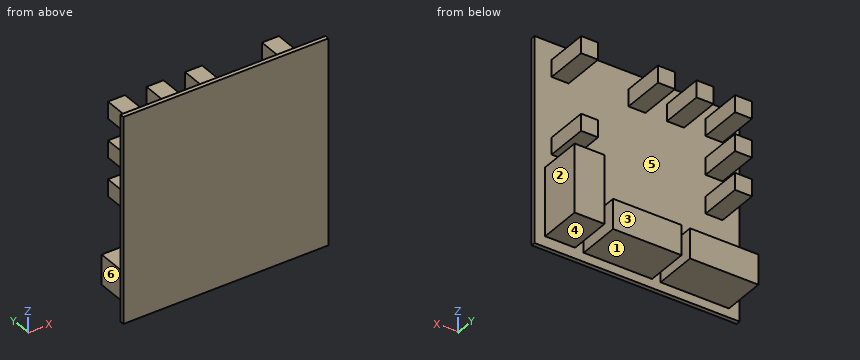
from build123d import *

# Parameters (mm, degrees)
SKETCH1_W              = 1.01
SKETCH1_H              = 1.01
BOSS_EXTRUDE1_DEPTH    = 2.54
BOSS_EXTRUDE1_2_DEPTH  = 2.54
BOSS_EXTRUDE1_3_DEPTH  = 2.54
BOSS_EXTRUDE1_4_DEPTH  = 2.54
BOSS_EXTRUDE1_5_DEPTH  = 2.54
BOSS_EXTRUDE1_6_DEPTH  = 2.54
BOSS_EXTRUDE1_7_DEPTH  = 2.54
SKETCH1_W_2            = 1.778
SKETCH1_H_2            = 4.064
BOSS_EXTRUDE1_8_DEPTH  = 2.54
SKETCH1_W_3            = 4.064
SKETCH1_H_3            = 1.778
BOSS_EXTRUDE1_9_DEPTH  = 2.54
BOSS_EXTRUDE1_10_DEPTH = 2.54
SKETCH3_W              = 12.192
SKETCH3_H              = 12.192
BOSS_EXTRUDE2_DEPTH    = 0.254


with BuildPart() as part:
    # Sketch1 (on Top Plane) → Boss-Extrude1 (new body)
    with BuildSketch(Plane(origin=(0, 0, 0), x_dir=(1, 0, 0), z_dir=(0, 1, 0))):
        with Locations((1.52, 1.52)):
            Rectangle(SKETCH1_W, SKETCH1_H)
    extrude(amount=BOSS_EXTRUDE1_DEPTH)



with BuildPart() as body_2:
    # Sketch1 (on Top Plane) → Boss-Extrude1 2 (new body)
    with BuildSketch(Plane(origin=(0, 0, 0), x_dir=(1, 0, 0), z_dir=(0, 1, 0))):
        with Locations((1.52, 6.096)):
            Rectangle(SKETCH1_W, SKETCH1_H)
    extrude(amount=BOSS_EXTRUDE1_2_DEPTH)


with BuildPart() as body_3:
    # Sketch1 (on Top Plane) → Boss-Extrude1 3 (new body)
    with BuildSketch(Plane(origin=(0, 0, 0), x_dir=(1, 0, 0), z_dir=(0, 1, 0))):
        with Locations((1.52, 3.81)):
            Rectangle(SKETCH1_W, SKETCH1_H)
    extrude(amount=BOSS_EXTRUDE1_3_DEPTH)


with BuildPart() as body_4:
    # Sketch1 (on Top Plane) → Boss-Extrude1 4 (new body)
    with BuildSketch(Plane(origin=(0, 0, 0), x_dir=(1, 0, 0), z_dir=(0, 1, 0))):
        with Locations((10.67, 1.52)):
            Rectangle(SKETCH1_W, SKETCH1_H)
    extrude(amount=BOSS_EXTRUDE1_4_DEPTH)


with BuildPart() as body_5:
    # Sketch1 (on Top Plane) → Boss-Extrude1 5 (new body)
    with BuildSketch(Plane(origin=(0, 0, 0), x_dir=(1, 0, 0), z_dir=(0, 1, 0))):
        with Locations((6.1, 1.52)):
            Rectangle(SKETCH1_W, SKETCH1_H)
    extrude(amount=BOSS_EXTRUDE1_5_DEPTH)


with BuildPart() as body_6:
    # Sketch1 (on Top Plane) → Boss-Extrude1 6 (new body)
    with BuildSketch(Plane(origin=(0, 0, 0), x_dir=(1, 0, 0), z_dir=(0, 1, 0))):
        with Locations((3.81, 1.52)):
            Rectangle(SKETCH1_W, SKETCH1_H)
    extrude(amount=BOSS_EXTRUDE1_6_DEPTH)


with BuildPart() as body_7:
    # Sketch1 (on Top Plane) → Boss-Extrude1 7 (new body)
    with BuildSketch(Plane(origin=(0, 0, 0), x_dir=(1, 0, 0), z_dir=(0, 1, 0))):
        with Locations((10.67, 6.096)):
            Rectangle(SKETCH1_W, SKETCH1_H)
    extrude(amount=BOSS_EXTRUDE1_7_DEPTH)


with BuildPart() as body_8:
    # Sketch1 (on Top Plane) → Boss-Extrude1 8 (new body)
    with BuildSketch(Plane(origin=(0, 0, 0), x_dir=(1, 0, 0), z_dir=(0, 1, 0))):
        with Locations((10.67, 9.525)):
            Rectangle(SKETCH1_W_2, SKETCH1_H_2)
    extrude(amount=BOSS_EXTRUDE1_8_DEPTH)


with BuildPart() as body_9:
    # Sketch1 (on Top Plane) → Boss-Extrude1 9 (new body)
    with BuildSketch(Plane(origin=(0, 0, 0), x_dir=(1, 0, 0), z_dir=(0, 1, 0))):
        with Locations((2.667, 10.769327267)):
            Rectangle(SKETCH1_W_3, SKETCH1_H_3)
    extrude(amount=BOSS_EXTRUDE1_9_DEPTH)


with BuildPart() as body_10:
    # Sketch1 (on Top Plane) → Boss-Extrude1 10 (new body)
    with BuildSketch(Plane(origin=(0, 0, 0), x_dir=(1, 0, 0), z_dir=(0, 1, 0))):
        with Locations((7.239, 10.769327267)):
            Rectangle(SKETCH1_W_3, SKETCH1_H_3)
    extrude(amount=BOSS_EXTRUDE1_10_DEPTH)


with BuildPart() as part_1:
    add(part.part)

    add(body_2.part)  # Boss-Extrude2 merges body 2

    add(body_3.part)  # Boss-Extrude2 merges body 3

    add(body_4.part)  # Boss-Extrude2 merges body 4

    add(body_5.part)  # Boss-Extrude2 merges body 5

    add(body_6.part)  # Boss-Extrude2 merges body 6

    add(body_7.part)  # Boss-Extrude2 merges body 7

    add(body_8.part)  # Boss-Extrude2 merges body 8

    add(body_9.part)  # Boss-Extrude2 merges body 9

    add(body_10.part)  # Boss-Extrude2 merges body 10
    # Sketch3 → Boss-Extrude2 (add)
    with BuildSketch(Plane.XZ):
        with Locations((6.096, -6.096)):
            Rectangle(SKETCH3_W, SKETCH3_H)
    extrude(amount=BOSS_EXTRUDE2_DEPTH)


solid = part_1.part
The model under review builds one solid part; all positions refer to its coordinate system, in mm. Face numbers are marked on the shaded views. A direction names the side the tool comes from. Round coordinates to 2 decimals unless told otherwise and drop trailing zeros. Loops run counter-clockwise (first coordinate to the right, second up) from the corner with the lowest first, then second, coordinate; pieces in that order, holes last. Notation, with made-up numbers: M -3.5,-1.75 L 2.5,-1.75 A17 cw 2.5,8.25 Z; hole C -15,9.25 d6. An arc over 180 degrees is marked long. Answer as CSV lines item,"result". Start each with the question number.
Item 1: Mouldability with a two-part tool opening along X and no side actions: class the marked faces 4, 5 and 6 as released by +X, released by -X, zero draft, split by the parting line, or undercut.
Item 2: Consider section B-B (x = 4.5). Write out the cut boundary in (y, z), then the cut area to 3 significant figures.
Item 3: For the marked faces 1, 2 and 3, list the 3-axis set-ups (+Z, -Z, +X, -X, +Y, -Y) from which the entire face can be reached by the end or side of a thin tool; tool diameter is ignored.
Item 4: Consider section D-D (z = -8). Write out the cut boundary in (x, y), then the cut area to 3 significant figures.
Item 5: Insertion check: P1, Ø1.1, axis at y = 1, z = -1.5, coming from the -X side (3 decimals); P2, Ø0.9, axis at y = 1.5, z = -10.5, coming from the -X side (3 decimals); P3, Ø0.5, axis at x = 1.5, y = 2, coming from the +Z side (3 decimals). Each pin has a flat end and moves straight along its axis. Give the tip position at first contact, or say it passes through.
Item 6: Consider section C-C (y = 1.35). State how many separate pieces and enclosed holes the cut face has, then the cut area to 3 significant figures.
Item 7: Wall thickness on line 1 (Z direction, x = 1.25, y = 2.3) (3 decimals); line 2 (X direction, y = 1.3, z = -10.25) (3 decimals); line 3 (X direction, y = 1.3, z = -1.5) (3 decimals): over which ranges is each line inside the solid? List them lowest first. Write a range as [from, to].
Item 8: Consider section A-A (z = -10.5). Write out the cut boundary in (x, y) (3 decimals).
Answer:
1,face 4,"zero draft"
1,face 5,"undercut"
1,face 6,"released by -X"
2,outline,"M -0.25,-12.19 L 0,-12.19 L 0,-11.66 L 2.54,-11.66 L 2.54,-9.88 L 0,-9.88 L 0,0 L -0.25,0 Z"
2,area,"7.61 mm^2"
3,face 1,"-Z, +X, -X, +Y"
3,face 2,"+Z, -Z, +X, +Y"
3,face 3,"+Z, -Z, +X, -X, +Y"
4,outline,"M 0,-0.25 L 12.19,-0.25 L 12.19,0 L 11.56,0 L 11.56,2.54 L 9.78,2.54 L 9.78,0 L 0,0 Z"
4,area,"7.61 mm^2"
5,P1,"stops at x = 1.015"
5,P2,"stops at x = 0.635"
5,P3,"stops at z = -1.015"
6,separate pieces,"10"
6,enclosed holes,"0"
6,area,"28.8 mm^2"
7,line 1,"z = [-11.658, -9.88], [-6.601, -5.591], [-4.315, -3.305], [-2.025, -1.015]"
7,line 2,"x = [0.635, 4.699], [5.207, 9.271], [9.781, 11.559]"
7,line 3,"x = [1.015, 2.025], [3.305, 4.315], [5.595, 6.605], [10.165, 11.175]"
8,outline,"M 0,-0.254 L 12.192,-0.254 L 12.192,0 L 11.559,0 L 11.559,2.54 L 9.781,2.54 L 9.781,0 L 9.271,0 L 9.271,2.54 L 5.207,2.54 L 5.207,0 L 4.699,0 L 4.699,2.54 L 0.635,2.54 L 0.635,0 L 0,0 Z"
